Geometry check sheet. Reference: the model listing, model coordinates, mm. Round coordinates to 2 decimals unless told otherwise and drop trailing zeros. Loops run counter-clockwise (first coordinate to the right, second up) from the corner with the lowest first, then second, coordinate; pieces in that order, holes last. Notation, with made-up numbers: (60.25, 2.5) -> (91.25, 2.5) arc R28 ccw to (91.25, 24.5) -> close; hole circle Ø1 at (-15.5, 70.25). An arc over 180 degrees is marked (long way). Use a Markdown table: item, result. Add a question column.
Q1. Material ranges on L1, parallel to Z at x = 47.25, y = 6.75; L2, parallel to Z at x = 41.75, y = 3; L3, parallel to Z at x = 31, y = 3, recorded low to high.
Q2. Gauge pin test, flat ends, axial feed: P1, Ø3, axis at x = 30.94, z = 11.48, coming from the -Y side; P2, Ø1, axis at y = 3, z = 13.5, coming from the +X side; P3, Ø2, axis at y = 3, z = 17.5, coming from the -X side. Record the tip position at first contact, or that the pin passes through.
Q3. Sectioned sample at B-B, the plane z = 17.75. Enter the section's corners in (x, y).
Q4. Sectioned sample at C-C, the plane x = 44.25. Enter the section's corners in (y, z).
Q5. Sectioned sample at A-A, the plane y = 3.25. Enter the section's corners in (x, z), then the cut area to 3 significant figures.
Q6. Release check for a two-part mould opening along Z. For faces 1 (the face through (40, 8, 16)), 2 (the face through (29.46, 4.67, 10.54)), 3 (the face through (49.72, 3.94, 18.35)) record: released by +Z, released by -Z, zero draft, split by the parting line, or undercut.
Autodesk Inventor part; units mm, degrees
ref_plane "YZ Plane" through (0, 0, 0) normal (1, 0, 0) x (0, 1, 0)
ref_plane "XZ Plane" through (0, 0, 0) normal (0, 1, 0) x (-1, 0, 0)
ref_plane "XY Plane" through (0, 0, 0) normal (0, 0, 1) x (1, 0, 0)
sketch "Sketch1" plane through (0, 0, 0) normal (0, 1, 0) x (-1, 0, 0)
  arc A0 (-33, 0) -> (-32.0949, 7.6757) centre (0, 0) ccw
  arc A1 (-40, 0) -> (-38.9029, 9.3039) centre (0, 0) ccw
  arc A2 (-53, 0) -> (-51.5464, 12.3276) centre (0, 0) ccw
  line L0 (-85, 0) -> (100, 0) construction
  line L1 (-226, 10) -> (0, 10) construction
  line L2 (0, 10) -> (0, -10) construction
  line L3 (0, -10) -> (-226, -10) construction
  line L4 (-226, -10) -> (-226, 10) construction
  line L5 (-226, 10) -> (0, -10) construction
  line L6 (0, 10) -> (-226, -10) construction
  line L7 (-52.0481, -10) -> (-44.1646, -51.032)
  line L8 (-38.9029, 9.3039) -> (-32.0949, 7.6757)
  line L9 (-52.0481, -10) -> (-84.6485, -16.2635)
  circle A3 centre (0, 0) radius 33 construction
  line L10 (0, 0) -> (-30.9399, 11.477) construction
  line L11 (-35.5594, 18.3175) -> (-29.3365, 15.1119)
  line L12 (-19.4128, 10) -> (0, 0)
  line L13 (0, 0) -> (-30.5202, 7.2991)
  line L14 (-32.0949, 7.6757) -> (-148.5747, 35.5325)
  line L15 (-35.5594, 18.3175) -> (-47.1162, 24.2707)
  point P0 (-113, 0)
  point P1 (-113, 0)
  point P2 (-45.9257, 26.4544)
  dimension "d13" = 66
  dimension "d0" = 66
  dimension "d1" = 80
  dimension "d2" = 106
  dimension "d3" = 20
  dimension "d5" = 100.876
  dimension "d11" = 90
  dimension "d12" = 10.876
extrude "Extrusion1" add sketch "Sketch1" along normal blind 10
sketch "Sketch3" plane through (0, 10, 0) normal (0, 1, 0) x (1, 0, 0)
  line L0 (29.3365, -15.1119) -> (47.1162, -24.2707)
  arc A0 (29.3365, -15.1119) -> (32.0949, -7.6757) centre (0, 0) ccw
  line L1 (51.5464, -12.3276) -> (32.0949, -7.6757)
  arc A1 (47.1162, -24.2707) -> (51.5464, -12.3276) centre (0, 0) ccw
  arc A2 (40, 0) -> (38.9029, -9.3039) centre (0, 0) ccw
  point P0 (35.5594, -18.3175)
extrude "Extrusion3" cut sketch "Sketch3" against normal blind 2
ref_plane "Work Plane1" through (30.9399, 0, 11.477) normal (0, -1, 0) x (-0.3478, 0, 0.9376)
sketch "Sketch5" plane through (0, 0, 0) normal (0, -1, 0) x (1, 0, 0)
  arc A0 (32.0949, 7.6757) -> (29.3365, 15.1119) centre (0, 0) ccw
  arc A1 (29.3365, 15.1119) -> (32.0949, 7.6757) centre (32.0126, 11.8749) ccw
  dimension "d38" = 4.2
extrude "Extrusion5" add sketch "Sketch5" against normal up to surface (8 mm away)
hole "Hole3" at (30.9399, 0, 11.477) direction (0, 1, 0) diameter 3.5 depth 8 tip angle 118 countersink diameter 6 countersink angle 90
equation "\"d13\" = d0"
equation "\"d15\" = 0.5 * d14"
properties part number "end_stop_plug_v3"
Values:
| question | item | result |
|---|---|---|
| 1 | L1 | 11.3 to 24.01 |
| 1 | L2 | 9.98 to 21.51 |
| 1 | L3 | 7.8 to 9.73, 13.23 to 15.97 |
| 2 | P1 | through |
| 2 | P2 | x = 51.38 |
| 2 | P3 | x = 32.03 |
| 3 | outline | (34.46, 0) -> (49.94, 0) -> (49.94, 8) -> (34.46, 8) -> close |
| 4 | outline | (0, 10.58) -> (8, 10.58) -> (8, 22.79) -> (0, 22.79) -> close |
| 5 | outline | (29.34, 15.11) arc R4.2 ccw to (32.09, 7.68) -> (38.9, 9.3) -> (51.55, 12.33) arc R53 ccw to (47.12, 24.27) -> (35.56, 18.32) -> close; hole circle Ø3.5 at (30.94, 11.48) |
| 5 | area | 215 mm^2 |
| 6 | face 1 | zero draft |
| 6 | face 2 | undercut |
| 6 | face 3 | released by +Z |
